Geometry check sheet. Reference: the model listing, model coordinates, mm. A direction names the side the tool comes from. Give positions to 0.01 mm unless a question says otherwise; leave off trailing zeros. Order: outer loops, then holes, each group sorted by start corner. A loop starts at its lowest first (then second) coordinate and runs counter-clockwise, first axis right, second up.
from build123d import *

# Parameters (mm, degrees)
BOSS_EXTRUDE4_DEPTH = 15
BOSS_EXTRUDE5_DEPTH = 5
BOSS_EXTRUDE8_DEPTH = 15
CUT_EXTRUDE2_DEPTH  = 10
BOSS_EXTRUDE9_DEPTH = 5
SKETCH11_R          = 5
CUT_EXTRUDE3_DEPTH  = 54
SKETCH12_R          = 5
SKETCH12_R_2        = 2.5
CUT_EXTRUDE4_DEPTH  = 76


with BuildPart() as part:
    # Sketch2 → Boss-Extrude4 (new body)
    with BuildSketch(Plane.XY):
        with BuildLine():
            Line((-55, 0), (0, 0))
            Line((0, 0), (0, 60))
            Line((0, 60), (-55, 60))
            ThreePointArc((-55, 60), (-85, 30), (-55, 0))
        make_face()
    extrude(amount=BOSS_EXTRUDE4_DEPTH)

    # Sketch5 → Boss-Extrude5 (add)
    with BuildSketch(Plane.XY.offset(15)):
        with BuildLine():
            Line((-84.047375097, 37.5), (-79.047375097, 37.5))
            ThreePointArc((-79.047375097, 37.5), (-69.870493007, 50.161897068), (-55, 55))
            Line((-55, 55), (-55, 60))
            ThreePointArc((-55, 60), (-73.371173071, 53.717082451), (-84.047375097, 37.5))
        make_face()
        with BuildLine():
            Line((-55, 0), (-55, 5))
            ThreePointArc((-55, 5), (-69.870493007, 9.838102932), (-79.047375097, 22.5))
            Line((-79.047375097, 22.5), (-84.047375097, 22.5))
            ThreePointArc((-84.047375097, 22.5), (-73.371173071, 6.282917549), (-55, 0))
        make_face()
    extrude(amount=BOSS_EXTRUDE5_DEPTH)

    # Sketch6 → Boss-Extrude8 (add)
    with BuildSketch(Plane.XY.offset(15)):
        with BuildLine():
            Line((-55, 60), (-55, 45))
            ThreePointArc((-55, 45), (-40, 30), (-55, 15))
            Line((-55, 15), (-55, 0))
            Line((-55, 0), (0, 0))
            Line((0, 0), (0, 60))
            Line((0, 60), (-55, 60))
        make_face()
    extrude(amount=BOSS_EXTRUDE8_DEPTH)

    # Sketch9 → Cut-Extrude2 (cut)
    with BuildSketch(Plane.XY.offset(30)):
        with BuildLine():
            Line((-43.819660113, 40), (0, 40))
            Line((0, 40), (0, 20))
            Line((0, 20), (-43.819660113, 20))
            ThreePointArc((-43.819660113, 20), (-40, 30), (-43.819660113, 40))
        make_face()
    extrude(amount=-CUT_EXTRUDE2_DEPTH, mode=Mode.SUBTRACT)

    # Sketch10 → Boss-Extrude9 (add)
    with BuildSketch(Plane.XY.offset(20)):
        with BuildLine():
            Line((-43.819660113, 40), (-21.319660113, 40))
            ThreePointArc((-21.319660113, 40), (-11.319660113, 30), (-21.319660113, 20))
            Line((-21.319660113, 20), (-43.819660113, 20))
            ThreePointArc((-43.819660113, 20), (-40, 30), (-43.819660113, 40))
        make_face()
    extrude(amount=BOSS_EXTRUDE9_DEPTH)

    # Sketch11 → Cut-Extrude3 (cut)
    with BuildSketch(Plane.XY.offset(25)):
        with Locations((-21.319660113, 30)):
            Circle(SKETCH11_R)
    extrude(amount=-CUT_EXTRUDE3_DEPTH, mode=Mode.SUBTRACT)

    # Sketch12 → Cut-Extrude4 (cut)
    with BuildSketch(Plane.XY.offset(15)):
        with Locations((-55, 30)):
            Circle(SKETCH12_R)
        with Locations((-65, 15)):
            Circle(SKETCH12_R_2)
        with Locations((-65, 45)):
            Circle(SKETCH12_R_2)
    extrude(amount=-CUT_EXTRUDE4_DEPTH, mode=Mode.SUBTRACT)


solid = part.part
Item 1: Sectioned sample at D-D (x = -38.5). Enter the section's corners in (y, z), and give its area (3 significant figures).
Reported:
outline: (0, 0) - (60, 0) - (60, 30) - (40, 30) - (40, 25) - (20, 25) - (20, 30) - (0, 30) - close
area: 1,700 mm2
Item 2: Sectioned sample at B-B (y = 30). Enter the section's corners in (x, z), and give its area (3 significant figures).
Reported:
outline: (-85, 0) - (-60, 0) - (-60, 15) - (-85, 15) - close; (-50, 0) - (-26.32, 0) - (-26.32, 25) - (-40, 25) - (-40, 15) - (-50, 15) - close; (-16.32, 0) - (0, 0) - (0, 20) - (-11.32, 20) - (-11.32, 25) - (-16.32, 25) - close
area: 1,220 mm2
Item 3: Scan lines: L1, parallel to Y at x = -65, z = 3.25; L2, parallel to Y at x = -55, z = 10; L3, parallel to Z at x = -70, y = 28. Record each from-to range of solid material in increasing order.
Reported:
L1: y = 1.72 to 12.5, 17.5 to 42.5, 47.5 to 58.28
L2: y = 0 to 25, 35 to 60
L3: z = 0 to 15
Item 4: Sectioned sample at A-A (z = 28.25). Enter the section's corners in (x, y), and give its area (3 significant figures).
Reported:
outline: (-55, 0) - (0, 0) - (0, 20) - (-43.82, 20) arc R15 cw to (-55, 15) - close; (-55, 45) arc R15 cw to (-43.82, 40) - (0, 40) - (0, 60) - (-55, 60) - close
area: 2,120 mm2
Item 5: Sectioned sample at C-C (z = 5.25). Enter the section's corners in (x, y).
Reported:
outline: (-55, 0) - (0, 0) - (0, 60) - (-55, 60) arc R30 ccw to start; hole circle Ø5 at (-65, 15); hole circle Ø5 at (-65, 45); hole circle Ø10 at (-55, 30); hole circle Ø10 at (-21.32, 30)
Item 6: Set-up check for faces 1 (the flat face through (-28, 50, 30)), 2 (the flat face through (-82, 22.5, 17)), 3 (the flat face through (-55, 53, 22)), 4 (the flat face through (-27, 30, 25)), 5 (the cylindrical face through (-62.69, 14.04, 7.6)): record each of +Z, -Z, +X, -X, +Y, -Y from which the full face is reachable in a straight line by a thin tool's end or side.
Reported:
face 1: +Z, +X, -X, +Y, -Y
face 2: +Z, -X
face 3: +Z
face 4: +Z, +X, -X
face 5: +Z, -Z
Item 7: Gauge pin test, flat ends, axial feed: pin 1 (7 mm diameter, centred on x = -65, y = 10, fed in from +Z); pin 2 (4 mm diameter, centred on x = -10.5, z = 17, fed in from -Y); pin 3 (16 mm diameter, centred on x = -10.5, y = 30, fed in from +Z); pin 4 (4 mm diameter, centred on x = -65, y = 15, fed in from +Z). Record the tip position at first contact, or that the pin passes through.
Reported:
pin 1: stops at z = 20
pin 2: stops at y = 0
pin 3: stops at z = 25
pin 4: passes through
Item 8: Draft check along X on faces 6 (the flat face through (-71, 50, 20)), 7 (the cylindrical face through (-62.69, 44.04, 7.6)), 8 (the flat face through (0, 30, 15)), 9 (the flat face through (-63, 30, 15)). Enter one of: released by +X, released by -X, zero draft, split by the parting line, or undercut.
Reported:
face 6: zero draft
face 7: undercut
face 8: released by +X
face 9: undercut
